Read the model definition and answer for the solid it produces. Units are mm, in the model's axes. A direction names the side the tool comes from. Coordinates: 2 decimals unless noted, no trailing zeros. Write each loop counter-clockwise with the first axis right and the second up, starting at its lowest first coordinate (ties: lowest second). Pieces come first, ordered by that corner, then holes. Notation, with made-up numbers: (87.5, 78.5) -> (130.5, 78.5) arc R28 ccw to (130.5, 103.5) -> close; hole circle Ø2 at (77.5, 2.25). An arc over 180 degrees is marked (long way). Answer in a Markdown table with one row per item. Add a question column.
Item 1: Section A-A on x = 12.7 is taken. Write down the section's boundary in (y, z).
Item 2: Section C-C on x = 23.5 is taken. Write down the section's boundary in (y, z), then the cut area to 3 significant figures.
Item 3: Section B-B on z = 1 is taken. Write down the section's boundary in (x, y), then the cut area to 3 significant figures.
Item 4: For a pull along X with two mould halves and no side action, classify faces 1 (the face through (25.4, 11.3, -5.6)), 2 (the face through (13, 11.112, -1)), 3 (the face through (0, 11.3, -5.6)), 4 (the face through (6.81, -2.21, -11.9)) as +X half, -X half, draft (parallel to the pull), parting line (faces both ways), or undercut.
Item 5: Section D-D on y = -9.5 is taken. Write down the section's boundary in (x, z), then the cut area to 3 significant figures.
Item 6: Straight lines are drawn through the part: line 1 (Z direction, x = 14.25, y = 1.5); line 2 (Y direction, x = 16.5, z = -6.25); line 3 (Y direction, x = 17.4, z = -12). For each, find the intervals that lie inside material, in ascending order. Write a range as from..to.
Item 7: Which of the six approach directions +Z, -Z, +X, -X, +Y, -Y give full straight-line access (tool end or side, diameter ignored) to faces 5 (the face through (12.522, 12.399, -12.415)), 6 (the face through (13, -1, -11.112))?
Item 8: Given pin 1 Ø4 at (x, y) = (17.4, -1.29) entering from +Z; pin 2 Ø11.5 at (x, z) = (12, 4.5) entering from -Y, each flat-ended and moving along its own axis, determine where each tip first touches the part or whether it passes through.
```python
from build123d import *

# Parameters (mm, degrees)
BOSS_EXTRUDE1_DEPTH = 25.4
SKETCH2_R           = 1.5
CUT_EXTRUDE1_DEPTH  = 25.4
SKETCH3_R           = 2.1
CUT_EXTRUDE2_DEPTH  = 25.4


with BuildPart() as part:
    # Sketch1 → Boss-Extrude1 (new body)
    with BuildSketch(Plane(origin=(0, 0, 0), x_dir=(0, 0, -1), z_dir=(1, 0, 0))):
        with BuildLine():
            Line((11.1125, -12.7), (12.7, -12.7))
            Line((12.7, -12.7), (12.7, 11.7))
            ThreePointArc((12.7, 11.7), (12.407106781, 12.407106781), (11.7, 12.7))
            Line((11.7, 12.7), (-12.7, 12.7))
            Line((-12.7, 12.7), (-12.7, 11.1125))
            Line((-12.7, 11.1125), (10.1125, 11.1125))
            ThreePointArc((10.1125, 11.1125), (10.819606781, 10.819606781), (11.1125, 10.1125))
            Line((11.1125, 10.1125), (11.1125, -12.7))
        make_face()
    extrude(amount=BOSS_EXTRUDE1_DEPTH)

    # Sketch2 → Cut-Extrude1 (cut)
    with BuildSketch(Plane.XY.offset(-11.1125)):
        with Locations((8, -1.29375)):
            Circle(SKETCH2_R)
        with Locations((17.4, -1.29375)):
            Circle(SKETCH2_R)
    extrude(amount=-CUT_EXTRUDE1_DEPTH, mode=Mode.SUBTRACT)

    # Sketch3 → Cut-Extrude2 (cut)
    with BuildSketch(Plane.XZ.offset(-11.1125)):
        with Locations(Location((12.7, 1.783154784, 0), (0, 0, 270))):
            Circle(SKETCH3_R)
    extrude(amount=-CUT_EXTRUDE2_DEPTH, mode=Mode.SUBTRACT)


solid = part.part
```
Results below:
| question | item | result |
|---|---|---|
| 1 | outline | (-12.7, -12.7) -> (11.7, -12.7) arc R1 ccw to (12.7, -11.7) -> (12.7, -0.32) -> (11.11, -0.32) -> (11.11, -10.11) arc R1 cw to (10.11, -11.11) -> (-12.7, -11.11) -> close; (11.11, 3.88) -> (12.7, 3.88) -> (12.7, 12.7) -> (11.11, 12.7) -> close |
| 2 | outline | (-12.7, -12.7) -> (11.7, -12.7) arc R1 ccw to (12.7, -11.7) -> (12.7, 12.7) -> (11.11, 12.7) -> (11.11, -10.11) arc R1 cw to (10.11, -11.11) -> (-12.7, -11.11) -> close |
| 2 | area | 78.1 mm2 |
| 3 | outline | (0, 11.11) -> (10.75, 11.11) -> (10.75, 12.7) -> (0, 12.7) -> close; (14.65, 11.11) -> (25.4, 11.11) -> (25.4, 12.7) -> (14.65, 12.7) -> close |
| 3 | area | 34.1 mm2 |
| 4 | face 1 | +X half |
| 4 | face 2 | draft |
| 4 | face 3 | -X half |
| 4 | face 4 | undercut |
| 5 | outline | (0, -12.7) -> (25.4, -12.7) -> (25.4, -11.11) -> (0, -11.11) -> close |
| 5 | area | 40.3 mm2 |
| 6 | line 1 | z = -12.7..-11.11 |
| 6 | line 2 | y = 11.11..12.7 |
| 6 | line 3 | y = -12.7..-2.79, 0.21..12.65 |
| 7 | face 5 | -Z, +X, -X, +Y |
| 7 | face 6 | +Z, +X, -X, -Y |
| 8 | pin 1 | stops at z = -11.11 |
| 8 | pin 2 | stops at y = 11.11 |
